Here's how the part is built. I have some questions about the finished solid (model axes, mm). A direction names the side the tool comes from. Coordinates: 2 decimals unless noted, no trailing zeros. Write each loop counter-clockwise with the first axis right and the second up, starting at its lowest first coordinate (ties: lowest second). Pieces come first, ordered by that corner, then holes. Notation, with made-up numbers: (-4, 44) - (21, 44) arc R14 cw to (21, 50) - close; hole circle Ø1 at (30, 74). An arc over 180 degrees is marked (long way). Answer in a Markdown table with one row per item. Add a question column.
Item 1: We'd pull the mould along X, two halves only. Please class faces 3 (the face through (-30, 0, 1)), 4 (the face through (23, 12, 1)), 5 (the face through (0, -5, 2.032)): +X half, -X half, draft (parallel to the pull), parting line (faces both ways), or undercut.
Item 2: Imagine slicing it at B-B (y = 9.5). Please give me the cut outline in (x, z), plus the area to 3 significant figures.
Item 3: Imagine slicing it at D-D (z = 0.75). State how many separate pieces and enclosed holes the cut face has, plus the area to 3 significant figures.
Item 4: I'm going to push a flat-ended pin straight in: pin 1 (4 mm diameter, centred on x = -19, y = 13, fed in from -Z). Where does the tip first touch, or does it pass through?
Item 5: Which directions (+Z, -Z, +X, -X, +Y, -Y) give clear straight access to the entire face, cutting with the end or side of a thin tool? Please do faces 1 (the face through (0, -5, 0)), 2 (the face through (25, 0.4, 1)).
Item 6: If I drill on probe 1 along Y at (x, z) = (-15, 1.5); probe 2 along Y at (x, z) = (-20, 1.3); probe 3 along Y at (x, z) = (-18, 0.85), over which ranges is the centre line in solid material (lowest first)? Write a range as from..to.
Item 7: Imagine slicing it at C-C (x = 2.5). Please give me the cut outline in (y, z).
Item 8: Imagine slicing it at A-A (x = 15). Please give me the cut outline in (y, z), plus the area to 3 significant figures.
from build123d import *

# Parameters (mm, degrees)
SKETCH1_W           = 60
SKETCH1_H           = 45
BOSS_EXTRUDE1_DEPTH = 2.032
FILLET1_R           = 5
SKETCH2_W           = 44.196
SKETCH2_H           = 23.114
CUT_EXTRUDE1_DEPTH  = 3.032
FILLET2_R           = 0.5
CUT_EXTRUDE2_DEPTH  = 3.032
SKETCH4_R           = 1.6
CUT_EXTRUDE3_DEPTH  = 3.032


with BuildPart() as part:
    # Sketch1 → Boss-Extrude1 (new body)
    with BuildSketch(Plane.XY):
        Rectangle(SKETCH1_W, SKETCH1_H)
    extrude(amount=BOSS_EXTRUDE1_DEPTH)

    # Fillet1
    fillet1_edges = [part.edges().sort_by_distance(p)[0] for p in [
        (30, -22.5, 1.016),
        (-30, -22.5, 1.016),
        (-30, 22.5, 1.016),
        (30, 22.5, 1.016),
    ]]
    fillet(fillet1_edges, radius=FILLET1_R)

    # Sketch2 → Cut-Extrude1 (cut, through all)
    with BuildSketch(Plane.XY.offset(2.032)):
        with Locations((0, 7.5)):
            Rectangle(SKETCH2_W, SKETCH2_H)
    extrude(amount=-CUT_EXTRUDE1_DEPTH, mode=Mode.SUBTRACT)

    # Fillet2
    fillet2_edges = [part.edges().sort_by_distance(p)[0] for p in [
        (22.098, 19.057, 1.016),
        (22.098, -4.057, 1.016),
        (-22.098, -4.057, 1.016),
        (-22.098, 19.057, 1.016),
    ]]
    fillet(fillet2_edges, radius=FILLET2_R)

    # Sketch3 → Cut-Extrude2 (cut, through all)
    with BuildSketch(Plane.XY.offset(2.032)):
        with BuildLine():
            ThreePointArc((-26.6, 13), (-25, 14.6), (-23.4, 13))
            Line((-23.4, 13), (-23.4, 12))
            ThreePointArc((-23.4, 12), (-25, 10.4), (-26.6, 12))
            Line((-26.6, 12), (-26.6, 13))
        make_face()
        with BuildLine():
            ThreePointArc((-26.6, 3), (-25, 4.6), (-23.4, 3))
            Line((-23.4, 3), (-22.098, 3))
            Line((-22.098, 3), (-22.098, 12))
            Line((-22.098, 12), (-23.4, 12))
            ThreePointArc((-23.4, 12), (-25, 10.4), (-26.6, 12))
            Line((-26.6, 12), (-26.6, 3))
        make_face()
        with BuildLine():
            Line((-26.6, 3), (-26.6, 2))
            ThreePointArc((-26.6, 2), (-25, 0.4), (-23.4, 2))
            Line((-23.4, 2), (-23.4, 3))
            ThreePointArc((-23.4, 3), (-25, 4.6), (-26.6, 3))
        make_face()
        with BuildLine():
            ThreePointArc((26.6, 2), (25, 0.4), (23.4, 2))
            Line((23.4, 2), (23.4, 3))
            ThreePointArc((23.4, 3), (25, 4.6), (26.6, 3))
            Line((26.6, 3), (26.6, 2))
        make_face()
        with BuildLine():
            ThreePointArc((23.4, 12), (25, 10.4), (26.6, 12))
            Line((26.6, 12), (26.6, 3))
            ThreePointArc((26.6, 3), (25, 4.6), (23.4, 3))
            Line((23.4, 3), (20.842092025, 3))
            Line((20.842092025, 3), (20.842092025, 12))
            Line((20.842092025, 12), (23.4, 12))
        make_face()
        with BuildLine():
            Line((26.6, 12), (26.6, 13))
            ThreePointArc((26.6, 13), (25, 14.6), (23.4, 13))
            Line((23.4, 13), (23.4, 12))
            ThreePointArc((23.4, 12), (25, 10.4), (26.6, 12))
        make_face()
    extrude(amount=-CUT_EXTRUDE2_DEPTH, mode=Mode.SUBTRACT)

    # Sketch4 → Cut-Extrude3 (cut, through all)
    with BuildSketch(Plane.XY.offset(2.032)):
        with Locations((-15, -15)):
            Circle(SKETCH4_R)
        with Locations((15, -15)):
            Circle(SKETCH4_R)
        with Locations((10, -17.5)):
            Circle(SKETCH4_R)
        with Locations((-10, -17.5)):
            Circle(SKETCH4_R)
        with Locations((20, -17.5)):
            Circle(SKETCH4_R)
        with Locations((-20, -17.5)):
            Circle(SKETCH4_R)
        with BuildLine():
            Line((1.6, -15), (1.6, -17.5))
            ThreePointArc((1.6, -17.5), (0, -19.1), (-1.6, -17.5))
            Line((-1.6, -17.5), (-1.6, -15))
            ThreePointArc((-1.6, -15), (0, -13.4), (1.6, -15))
        make_face()
    extrude(amount=-CUT_EXTRUDE3_DEPTH, mode=Mode.SUBTRACT)


solid = part.part
Here are the results:
| question | item | result |
|---|---|---|
| 1 | face 3 | -X half |
| 1 | face 4 | undercut |
| 1 | face 5 | draft |
| 2 | outline | (-30, 0) - (-26.6, 0) - (-26.6, 2.03) - (-30, 2.03) - close; (26.6, 0) - (30, 0) - (30, 2.03) - (26.6, 2.03) - close |
| 2 | area | 13.8 mm2 |
| 3 | separate pieces | 1 |
| 3 | enclosed holes | 8 |
| 3 | area | 1,480 mm2 |
| 4 | pin 1 | passes through |
| 5 | face 1 | -Z, +X, -X, +Y, -Y |
| 5 | face 2 | +Z, -Z |
| 6 | probe 1 | y = -22.5..-16.6, -13.4..-4.06, 19.06..22.5 |
| 6 | probe 2 | y = -22.5..-19.1, -15.9..-4.06, 19.06..22.5 |
| 6 | probe 3 | y = -22.5..-4.06, 19.06..22.5 |
| 7 | outline | (-22.5, 0) - (-4.06, 0) - (-4.06, 2.03) - (-22.5, 2.03) - close; (19.06, 0) - (22.5, 0) - (22.5, 2.03) - (19.06, 2.03) - close |
| 8 | outline | (-22.5, 0) - (-16.6, 0) - (-16.6, 2.03) - (-22.5, 2.03) - close; (-13.4, 0) - (-4.06, 0) - (-4.06, 2.03) - (-13.4, 2.03) - close; (19.06, 0) - (22.5, 0) - (22.5, 2.03) - (19.06, 2.03) - close |
| 8 | area | 38.0 mm2 |
